Input: part model. Units: mm. Frame: model coordinates. Coordinates: 2 decimals unless noted, no trailing zeros. Write each loop counter-clockwise with the first axis right and the second up, starting at its lowest first coordinate (ties: lowest second). Pieces come first, ordered by that corner, then holes. Notation, with made-up numbers: (-12.5, 86.25) -> (2.5, 86.25) arc R32 cw to (2.5, 115.25) -> close; hole circle Ø4 at (-6.75, -9.5). An arc over 180 degrees is marked (long way). Use one line per item in the form item = value. Start each with the question number.
(1) Ray query, line 1 along Y through (x, z) = (-16.5, 26); line 2 along Z through (x, y) = (-31, 0.15); line 3 along Z through (x, y) = (-28, -0.1). Return the intervals inside material, ascending.
(2) Cut plane A-A on x = -22. Return the cut outline in (y, z).
(3) Cut plane C-C on z = 39. Return the cut outline in (x, y).
(4) First-contact query: pin 1 (1.5 mm diameter, centred on x = -32.4, z = 28.84, fed in from -Y); pin 2 (0.6 mm diameter, centred on x = -31, z = 27.5, fed in from -Y); pin 3 (1.5 mm diameter, centred on x = -30.86, z = 29.48, fed in from +Y); pin 4 (2 mm diameter, centred on x = -36, z = 26, fed in from -Y) (3 decimals). Flat tips, straight axial feed; report the tip coordinate or a pass-through.
(5) Cut plane B-B on y = 0.55. Return the cut outline in (x, z) (3 decimals), plus the area to 3 significant figures.
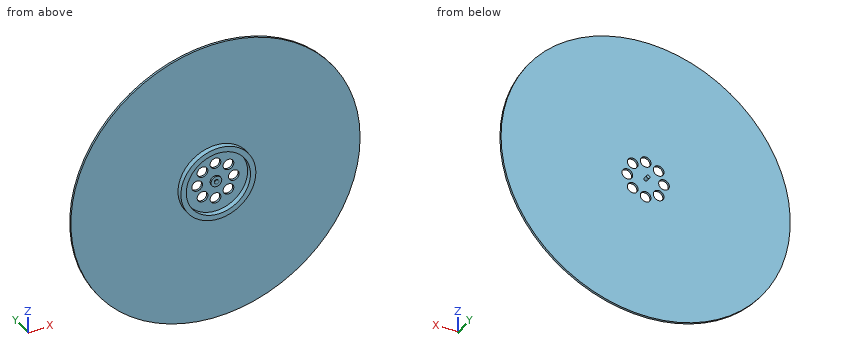
```python
from build123d import *

# Parameters (mm, degrees)
F0_R      = 17.145
F1_DEPTH  = 0.254
F2_R      = 4.445
F2_R_2    = 3.81
F3_DEPTH  = 0.635
F4_R      = 0.635
F5_DEPTH  = 0.2032
F6_R      = 0.254
F7_DEPTH  = 0.09398
F8_R      = 0.635
F9_DEPTH  = 1.8796
F10_R     = 0.2032
F11_DEPTH = 0.5588


with BuildPart() as f1:
    # F0 (on Front) → F1 (new body)
    with BuildSketch(Plane.XZ):
        with Locations((-30.861, 27.305001)):
            Circle(F0_R)
    extrude(amount=-F1_DEPTH)

    # F2 (on Front) → F3 (join)
    with BuildSketch(Plane.XZ):
        with Locations((-30.861057, 27.305188)):
            Circle(F2_R)
        with Locations((-30.861057, 27.305188)):
            Circle(F2_R_2, mode=Mode.SUBTRACT)
    extrude(amount=F3_DEPTH)

    # F4 (on face) → F5 (join)
    with BuildSketch(Plane.XZ):
        with Locations((-30.861109, 27.30538)):
            Circle(F4_R)
    extrude(amount=F5_DEPTH)

    # F6 (on face) → F7 (join)
    with BuildSketch(Plane.XZ.offset(0.2032)):
        with Locations((-30.861109, 27.30538)):
            Circle(F6_R)
    extrude(amount=F7_DEPTH)

    # F8 (on face) → F9 (cut)
    with BuildSketch(Plane.XZ.offset(0.635)):
        with Locations((-30.864747, 29.480701)):
            Circle(F8_R)
        with Locations((-29.325346, 28.846117)):
            Circle(F8_R)
        with Locations((-28.685544, 27.308878)):
            Circle(F8_R)
        with Locations((-29.320128, 25.769476)):
            Circle(F8_R)
        with Locations((-30.857367, 25.129674)):
            Circle(F8_R)
        with Locations((-33.036571, 27.301498)):
            Circle(F8_R)
        with Locations((-32.401987, 28.840899)):
            Circle(F8_R)
        with Locations((-32.396769, 25.764258)):
            Circle(F8_R)
    extrude(amount=-F9_DEPTH, mode=Mode.SUBTRACT)

    # F10 (on face) → F11 (join)
    with BuildSketch(Plane(origin=(0, 0.254, 0), x_dir=(-1, 0, 0), z_dir=(0, 1, 0))):
        with Locations((30.861, 27.305001)):
            Circle(F10_R)
    extrude(amount=F11_DEPTH)


solid = f1.part
```
Values:
q1.line_1 = 0 to 0.25
q1.line_2 = 10.16 to 24.51, 25.75 to 28.86, 30.1 to 44.45
q1.line_3 = 23.9 to 24.79, 29.82 to 30.71
q2.outline = (0, 12.63) -> (0.25, 12.63) -> (0.25, 41.98) -> (0, 41.98) -> close
q3.outline = (-43.4, 0) -> (-18.32, 0) -> (-18.32, 0.25) -> (-43.4, 0.25) -> close
q4.pin_1 = 0
q4.pin_2 = -0.3
q4.pin_3 = 0.25
q4.pin_4 = -0.635
q5.outline = circle Ø0.406 at (-30.861, 27.305)
q5.area = 0.130 mm2
